```python
from build123d import *

# Parameters (mm, degrees)
F0_W     = 60
F0_H     = 40
F1_DEPTH = 10
F3_DEPTH = 20
F4_R     = 10
F5_DEPTH = 25


with BuildPart() as f1:
    # F0 (on Top) → F1 (new body)
    with BuildSketch(Plane.XY):
        with Locations((30, 20)):
            Rectangle(F0_W, F0_H)
    extrude(amount=F1_DEPTH)

    # F2 (on face) → F3 (join)
    with BuildSketch(Plane.XZ):
        with BuildLine():
            Line((54.994119, 20), (40, 20))
            ThreePointArc((40, 20), (20, 40), (0, 20))
            Line((0, 20), (0, 10))
            Line((0, 10), (60, 10))
            Line((60, 10), (59.994116, 15.005877))
            ThreePointArc((59.994116, 15.005877), (58.527575, 18.537611), (54.994119, 20))
        make_face()
    extrude(amount=-F3_DEPTH)

    # F4 (on Front) → F5 (cut)
    with BuildSketch(Plane.XZ):
        with Locations((19.999131, 20.18641)):
            Circle(F4_R)
    extrude(amount=-F5_DEPTH, mode=Mode.SUBTRACT)


solid = f1.part
```
CAD build for the part. Positions are in the model's coordinates, mm. A direction names the side the tool comes from. Coordinates: 2 decimals unless noted, no trailing zeros. Order: outer loops, then holes, each group sorted by start corner. A loop starts at its lowest first (then second) coordinate and runs counter-clockwise, first axis right, second up. Notation, with made-up numbers: (51.5, 37) - (83.5, 37) arc R24 cw to (83.5, 67) - close; hole circle Ø5 at (80, -24.75). An arc over 180 degrees is marked (long way). Answer in a Markdown table with one row per item.
1. Drill centre lines: L1, parallel to X at y = 11, z = 11; L2, parallel to X at y = 17, z = 12.5; L3, parallel to Y at x = 42, z = 18. Where is each one in solid material? Low to high. Write a range as from..to.
Answer:
| item | result |
|---|---|
| L1 | 0..16.05, 23.95..60 |
| L2 | 0..13.6, 26.4..60 |
| L3 | 0..20 |
2. Pull direction Z, two halves, no side cores. Call faces 4 (the face through (18.7, 9.9, 30.1)), 5 (the face through (30, 0, 16)), 6 (the face through (30, 20, 0)), 7 (the face through (20, 10, 40)): +Z half, -Z half, draft (parallel to the pull), parting line (faces both ways), or undercut.
Answer:
| item | result |
|---|---|
| face 4 | undercut |
| face 5 | draft |
| face 6 | -Z half |
| face 7 | +Z half |
3. Slice it at A-A, the plane x = 20. List the corners of the cut face in (y, z), then the cut area to 3 significant figures.
Answer:
| item | result |
|---|---|
| outline | (0, 0) - (40, 0) - (40, 10) - (20, 10) - (20, 10.19) - (0, 10.19) - close; (0, 30.19) - (20, 30.19) - (20, 40) - (0, 40) - close |
| area | 600 mm² |
4. 3-axis set-ups, long thin cutter, end or side, ignore diameter. For faces 1 (the face through (30, 20, 25)), 2 (the face through (48, 10, 20)), 3 (the face through (0, 15, 8)): which of +Z, -Z, +X, -X, +Y, -Y reach the whole face in a straight line?
Answer:
| item | result |
|---|---|
| face 1 | +Z, +X, -X, +Y |
| face 2 | +Z, +X, +Y, -Y |
| face 3 | +Z, -Z, -X, +Y, -Y |
5. Slice it at D-D, the plane x = 53. List the corners of the cut face in (y, z).
Answer:
| item | result |
|---|---|
| outline | (0, 0) - (40, 0) - (40, 10) - (20, 10) - (20, 20) - (0, 20) - close |
6. Slice it at B-B, the plane z = 12.5. List the corners of the cut face in (x, y).
Answer:
| item | result |
|---|---|
| outline | (0, 0) - (13.6, 0) - (13.6, 20) - (0, 20) - close; (26.4, 0) - (60, 0) - (60, 20) - (26.4, 20) - close |
7. Flat gauge pins, fed straight in: P1, Ø2, axis at x = 28.5, y = 33, coming from the +Z side; P2, Ø5, axis at y = 23.5, z = 13.5, coming from the -X side; P3, Ø12, axis at x = 7, y = 4, coming from the -Z side; P4, Ø10, axis at y = 10.5, z = 26.5, coming from the -X side. Where does each tip first touch, or does it go through?
Answer:
| item | result |
|---|---|
| P1 | z = 10 |
| P2 | through |
| P3 | z = 0 |
| P4 | x = 0.06 |
8. Slice it at C-C, the plane y = 14. List the corners of the cut face in (x, z).
Answer:
| item | result |
|---|---|
| outline | (0, 0) - (60, 0) - (60, 10) - (59.99, 15.01) arc R5 ccw to (54.99, 20) - (40, 20) arc R20 ccw to (0, 20) - close; hole circle Ø20 at (20, 20.19) |
